from build123d import *

# Parameters (mm, degrees)
SKETCH1_W           = 101.6
SKETCH1_H           = 59.69
BOSS_EXTRUDE1_DEPTH = 2.3622
CUT_EXTRUDE1_REACH  = 4.362
SKETCH2_R           = 1.4
SKETCH2_R_2         = 2
SKETCH2_R_3         = 2.876999961
SKETCH4_W           = 2.4892
SKETCH4_H           = 9.525
CUT_EXTRUDE3_DEPTH  = 3.3622


with BuildPart() as part:
    # Sketch1 → Boss-Extrude1 (new body)
    with BuildSketch(Plane(origin=(0, 0, 0), x_dir=(0, 0, -1), z_dir=(1, 0, 0))):
        with Locations((50.8, 29.845)):
            Rectangle(SKETCH1_W, SKETCH1_H)
    extrude(amount=BOSS_EXTRUDE1_DEPTH)

    # Sketch2 → Cut-Extrude1 (cut, up to next)
    with BuildSketch(Plane(origin=(2.3622, 0, 0), x_dir=(0, 0, -1), z_dir=(1, 0, 0)), mode=Mode.PRIVATE) as cut_extrude1_sk1:
        with Locations((30.59102, 10.3)):
            Circle(SKETCH2_R)
    cut_extrude1_tool1 = extrude(cut_extrude1_sk1.sketch, amount=-CUT_EXTRUDE1_REACH, mode=Mode.PRIVATE) & part.part
    add(cut_extrude1_tool1.solids().sort_by_distance((2.3622, 10.3, -30.59102))[0], mode=Mode.SUBTRACT)
    # Sketch2 → Cut-Extrude1 (cut, up to next)
    with BuildSketch(Plane(origin=(2.3622, 0, 0), x_dir=(0, 0, -1), z_dir=(1, 0, 0)), mode=Mode.PRIVATE) as cut_extrude1_sk2:
        with Locations((30.59102, 27.8)):
            Circle(SKETCH2_R)
    cut_extrude1_tool2 = extrude(cut_extrude1_sk2.sketch, amount=-CUT_EXTRUDE1_REACH, mode=Mode.PRIVATE) & part.part
    add(cut_extrude1_tool2.solids().sort_by_distance((2.3622, 27.8, -30.59102))[0], mode=Mode.SUBTRACT)
    # Sketch2 → Cut-Extrude1 (cut, up to next)
    with BuildSketch(Plane(origin=(2.3622, 0, 0), x_dir=(0, 0, -1), z_dir=(1, 0, 0)), mode=Mode.PRIVATE) as cut_extrude1_sk3:
        with Locations((22.0000034, 19.05)):
            Circle(SKETCH2_R_2)
    cut_extrude1_tool3 = extrude(cut_extrude1_sk3.sketch, amount=-CUT_EXTRUDE1_REACH, mode=Mode.PRIVATE) & part.part
    add(cut_extrude1_tool3.solids().sort_by_distance((2.3622, 19.05, -22.000003))[0], mode=Mode.SUBTRACT)
    # Sketch2 → Cut-Extrude1 (cut, up to next)
    with BuildSketch(Plane(origin=(2.3622, 0, 0), x_dir=(0, 0, -1), z_dir=(1, 0, 0)), mode=Mode.PRIVATE) as cut_extrude1_sk4:
        with Locations((11, 19.05)):
            Circle(SKETCH2_R_3)
    cut_extrude1_tool4 = extrude(cut_extrude1_sk4.sketch, amount=-CUT_EXTRUDE1_REACH, mode=Mode.PRIVATE) & part.part
    add(cut_extrude1_tool4.solids().sort_by_distance((2.3622, 19.05, -11))[0], mode=Mode.SUBTRACT)

    # Sketch4 → Cut-Extrude3 (cut, through all)
    with BuildSketch(Plane(origin=(2.3622, 0, 0), x_dir=(0, 0, -1), z_dir=(1, 0, 0))):
        with Locations((7.5946, 45.3517)):
            Rectangle(SKETCH4_W, SKETCH4_H)
        with Locations((94.0054, 45.3517)):
            Rectangle(SKETCH4_W, SKETCH4_H)
    extrude(amount=-CUT_EXTRUDE3_DEPTH, mode=Mode.SUBTRACT)


solid = part.part
The listing builds one solid part. Answer for the finished solid, in the listing's coordinates (mm). A direction names the side the tool comes from. Coordinates: 2 decimals unless noted, no trailing zeros. Order: outer loops, then holes, each group sorted by start corner. A loop starts at its lowest first (then second) coordinate and runs counter-clockwise, first axis right, second up. Notation, with made-up numbers: M 34.25,-29 L 42.25,-29 A17 cw 42.25,-8 Z; hole C 17,72.25 d5. An arc over 180 degrees is marked long. Use CSV: the item, a comma, the result in double quotes.
Q1. Straight lines are drawn through the part: L1, parallel to Z at x = 0.1, y = 44; L2, parallel to Y at x = 0.6, z = -11; L3, parallel to Z at x = 1.4, y = 10. For each, find the intervals that lie inside material, in ascending order.
Here are the results:
L1,"-101.6 to -95.25, -92.76 to -8.84, -6.35 to 0"
L2,"0 to 16.17, 21.93 to 59.69"
L3,"-101.6 to -31.96, -29.22 to 0"
Q2. A tool of negligible diameter and unlimited length cuts with its end or side. For faces 4 (the flat face through (1, 59.69, -50)), 5 (the flat face through (1, 45, -95.25)), from which of +Z, -Z, +X, -X, +Y, -Y can it reach the whole face along a straight path? Write none if from no direction.
Here are the results:
face 4,"+Z, -Z, +X, -X, +Y"
face 5,"+X, -X"
Q3. Section D-D (y = 19.05) is taken. Determine the outline of the cut face in (x, z), then the cut area to 3 significant figures.
Here are the results:
outline,"M 0,-101.6 L 2.36,-101.6 L 2.36,-24 L 0,-24 Z; M 0,-20 L 2.36,-20 L 2.36,-13.88 L 0,-13.88 Z; M 0,-8.12 L 2.36,-8.12 L 2.36,0 L 0,0 Z"
area,"217 mm2"
Q4. Given pin 1 Ø3 at (y, z) = (27.8, -30.59) entering from -X, flat-ended and moving along its own axis, determine where the tip first touches the part or whether it passes through.
Here are the results:
pin 1,"x = 0"
Q5. Section B-B (z = -11) is taken. Determine the outline of the cut face in (x, y).
Here are the results:
outline,"M 0,0 L 2.36,0 L 2.36,16.17 L 0,16.17 Z; M 0,21.93 L 2.36,21.93 L 2.36,59.69 L 0,59.69 Z"
Q6. Section A-A (y = 27.8) is taken. Determine the outline of the cut face in (x, z), then the cut area to 3 significant figures.
Here are the results:
outline,"M 0,-101.6 L 2.36,-101.6 L 2.36,-31.99 L 0,-31.99 Z; M 0,-29.19 L 2.36,-29.19 L 2.36,0 L 0,0 Z"
area,"233 mm2"
Q7. Determine the mould class of faces 1 (the flat face through (1, 45, -6.35)), 2 (the flat face through (2.362, 30, -50)), 3 (the flat face through (1, 29, 0)) for opening direction Z: pulls with the +Z half, pulls with the -Z half, needs draft (parallel to the pull), parting line crosses it, or undercut.
Here are the results:
face 1,"undercut"
face 2,"needs draft"
face 3,"pulls with the +Z half"
Q8. Section C-C (x = 1.5) is taken. Determine the outline of the cut face in (y, z), then the cut area to 3 significant figures.
Here are the results:
outline,"M 0,-101.6 L 59.69,-101.6 L 59.69,0 L 0,0 Z; hole C 10.3,-30.59 d2.8; hole C 19.05,-11 d5.75; hole C 19.05,-22 d4; hole C 27.8,-30.59 d2.8; hole M 40.59,-95.25 L 50.11,-95.25 L 50.11,-92.76 L 40.59,-92.76 Z; hole M 40.59,-8.84 L 50.11,-8.84 L 50.11,-6.35 L 40.59,-6.35 Z"
area,"5,970 mm2"
